Design review of the part shown in the three views and the two pictorial views. Dimensions are in mm from the part's minimum x, y and z. A direction names the side the tool comes from. Round coordinates to 2 decimals unless told otherwise and drop trailing zeros. Write each loop counter-clockwise with the first axis right and the second up, starting at its lowest first coordinate (ties: lowest second). Pieces come first, ordered by that corner, then holes. Notation, with made-up numbers: (-12, -36) - (14, -36) arc R31 ccw to (14, -6) - close; hole circle Ø5 at (79, 57). An arc over 180 degrees is marked (long way). One line per item, written item: value. Start each with the question number.
Q1. Clearance check with flat-ended pins moving along their axes: pin 1 Ø2 at (x, y) = (1, 1.5) entering from -Z; pin 2 Ø3 at (y, z) = (1, 12) entering from +X; pin 3 Ø1 at (y, z) = (4.5, 5.5) entering from -X. State where each tip first meets the part, or that it passes through.
Q2. Add section D-D on y = 0.7. Write out the cut boundary in (x, z), and give its area (3 significant figures).
Q3. For probe 1 along Z at (x, y) = (0.95, 3.8); probe 2 along X at (y, z) = (4.05, 13.5); probe 3 along Y at (x, z) = (5.45, 4.5), list the stretches that pass through material, from the lowest coordinate up.
Q4. Tool access review of the marked faces 1 and 2: name each direction out of +Z, -Z, +X, -X, +Y, -Y from which nothing blocks a thin tool from reaching the whole face with its end or side.
Q5. Add section C-C on z = 8.75. Write out the cut boundary in (x, y), and give its area (3 significant figures).
Q6. Add section A-A on y = 2.95. Write out the cut boundary in (x, z), and give its area (3 significant figures).
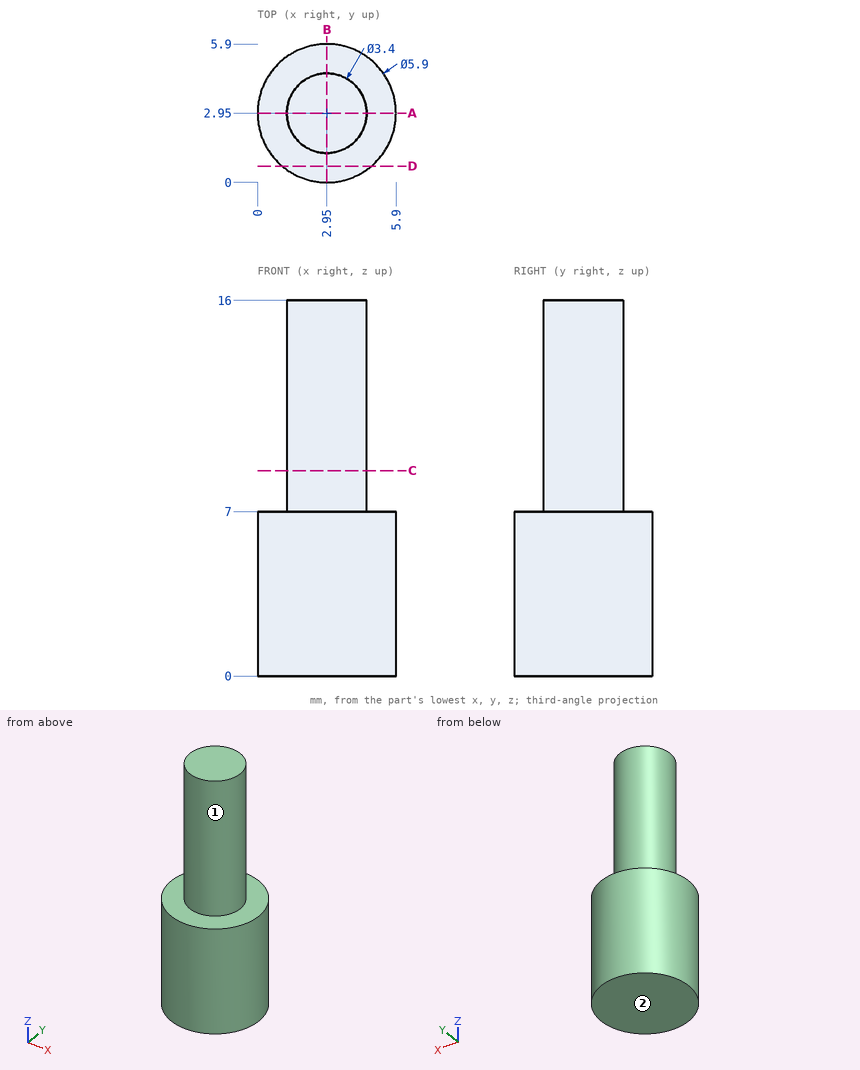
Result set:
1. pin 1: stops at z = 0
1. pin 2: stops at x = 4.59
1. pin 3: stops at x = 0.19
2. outline: (1.04, 0) - (4.86, 0) - (4.86, 7) - (1.04, 7) - close
2. area: 26.7 mm^2
3. probe 1: z = 0 to 7
3. probe 2: x = 1.65 to 4.25
3. probe 3: y = 1.38 to 4.52
4. face 1: +Z
4. face 2: -Z, +X, -X, +Y, -Y
5. outline: circle Ø3.4 at (2.95, 2.95)
5. area: 9.08 mm^2
6. outline: (0, 0) - (5.9, 0) - (5.9, 7) - (4.65, 7) - (4.65, 16) - (1.25, 16) - (1.25, 7) - (0, 7) - close
6. area: 71.9 mm^2
